For this review, take the finished solid that the model builds, in its own axes (mm). Coordinates: 2 decimals unless noted, no trailing zeros. Write each loop counter-clockwise with the first axis right and the second up, starting at its lowest first coordinate (ties: lowest second). Pieces come first, ordered by that corner, then holes. Notation, with made-up numbers: M 37.5,-4 L 48.5,-4 A14 cw 48.5,2 Z; hole C 49,-20 d4. An arc over 180 degrees is marked long. Return JSON: item names as keys, results as strings.
Autodesk Inventor part; units mm, degrees
ref_plane "YZ Plane" through (0, 0, 0) normal (1, 0, 0) x (0, 1, 0)
ref_plane "XZ Plane" through (0, 0, 0) normal (0, 1, 0) x (-1, 0, 0)
ref_plane "XY Plane" through (0, 0, 0) normal (0, 0, 1) x (1, 0, 0)
sketch "Sketch1" plane through (0, 0, 0) normal (0, 0, 1) x (1, 0, 0)
  line L0 (-52.5, -60) -> (52.5, -60)
  line L1 (52.5, -60) -> (52.5, 60)
  line L2 (52.5, 60) -> (-52.5, 60)
  line L3 (-52.5, 60) -> (-52.5, -60)
  line L4 (-52.5, -60) -> (52.5, 60) construction
  line L5 (52.5, -60) -> (-52.5, 60) construction
  point P0 (0, 0)
  dimension "d0" = 105
  dimension "d1" = 120
extrude "Extrusion1" add sketch "Sketch1" along normal blind 3
sketch "Sketch2" plane through (0, 0, 3) normal (0, 0, 1) x (1, 0, 0)
  circle A0 centre (-47, 55) radius 1.75
  line L0 (-73.5, 0) -> (73.5, 0) construction
  line L1 (0, 84) -> (0, -84) construction
  circle A1 centre (47, 55) radius 1.75
  circle A2 centre (-47, -55) radius 1.75
  circle A3 centre (47, -55) radius 1.75
  point P0 (0, 0)
  dimension "d4" = 3.5
  dimension "d5" = 94
  dimension "d6" = 110
extrude "Extrusion2" cut sketch "Sketch2" against normal blind 3
sketch "Sketch3" plane through (0, 0, 3) normal (0, 0, 1) x (1, 0, 0)
  line L0 (52.5, 60) -> (-52.5, 60) construction
  line L1 (52.5, 60) -> (-52.5, 60) construction
  line L2 (-41, 60) -> (41, 60)
  line L3 (41, 60) -> (41, 15)
  line L4 (41, 15) -> (-41, 15)
  line L5 (-41, 15) -> (-41, 60)
  line L6 (-52.5, 60) -> (-52.5, -60) construction
  line L7 (52.5, -60) -> (52.5, 60) construction
  line L8 (-73.5, 0) -> (73.5, 0)
  line L9 (52.5, -60) -> (-52.5, -60) construction
  line L10 (52.5, -60) -> (-52.5, -60) construction
  line L11 (-41, -60) -> (41, -60)
  line L12 (41, -60) -> (41, -15)
  line L13 (41, -15) -> (-41, -15)
  line L14 (-41, -15) -> (-41, -60)
  point P0 (0, 0)
  dimension "d9" = 15
  dimension "d10" = 82
  dimension "d11" = 11.5
  dimension "d12" = 105
extrude "Extrusion3" cut sketch "Sketch3" against normal blind 3
fillet "Fillet1" radius 2 4 edges at (-41, 15, 1.5) (41, 15, 1.5) (41, -15, 1.5) (-41, -15, 1.5)
fillet "Fillet2" radius 2 8 edges at (41, 60, 1.5) (52.5, 60, 1.5) (-41, 60, 1.5) (-52.5, 60, 1.5) (-52.5, -60, 1.5) (-41, -60, 1.5) (41, -60, 1.5) (52.5, -60, 1.5)
chamfer "Chamfer1" distance 0.75 angle 45 24 edges at (52.5, 0, 3) (51.9142, 59.4142, 3) (46.75, 60, 3) (41.5858, 59.4142, 3) (41, 37.5, 3) (40.4142, 15.5858, 3) (0, 15, 3) (-40.4142, 15.5858, 3) (-41, 37.5, 3) (-41.5858, 59.4142, 3) (-46.75, 60, 3) (-51.9142, 59.4142, 3) (-52.5, 0, 3) (-51.9142, -59.4142, 3) (-46.75, -60, 3) (-41.5858, -59.4142, 3) (-41, -37.5, 3) (-40.4142, -15.5858, 3) (0, -15, 3) (40.4142, -15.5858, 3) (41, -37.5, 3) (41.5858, -59.4142, 3) (46.75, -60, 3) (51.9142, -59.4142, 3)
sketch "Sketch4" plane through (0, 0, 3) normal (0, 0, 1) x (1, 0, 0)
  line L0 (-41, 17) -> (-41, 58)
  arc A0 (-41, 17) -> (-39, 15) centre (-39, 17) ccw
  line L1 (39, 15) -> (-39, 15)
  arc A1 (39, 15) -> (41, 17) centre (39, 17) ccw
  line L2 (41, 58) -> (41, 17)
  arc A2 (43, 60) -> (41, 58) centre (43, 58) ccw
  line L3 (50.5, 60) -> (43, 60)
  arc A3 (52.5, 58) -> (50.5, 60) centre (50.5, 58) ccw
  line L4 (52.5, -58) -> (52.5, 58)
  arc A4 (50.5, -60) -> (52.5, -58) centre (50.5, -58) ccw
  line L5 (43, -60) -> (50.5, -60)
  arc A5 (41, -58) -> (43, -60) centre (43, -58) ccw
  line L6 (41, -17) -> (41, -58)
  arc A6 (41, -17) -> (39, -15) centre (39, -17) ccw
  line L7 (-39, -15) -> (39, -15)
  arc A7 (-39, -15) -> (-41, -17) centre (-39, -17) ccw
  line L8 (-41, -58) -> (-41, -17)
  arc A8 (-43, -60) -> (-41, -58) centre (-43, -58) ccw
  line L9 (-50.5, -60) -> (-43, -60)
  arc A9 (-52.5, -58) -> (-50.5, -60) centre (-50.5, -58) ccw
  line L10 (-52.5, 58) -> (-52.5, -58)
  arc A10 (-50.5, 60) -> (-52.5, 58) centre (-50.5, 58) ccw
  line L11 (-43, 60) -> (-50.5, 60)
  arc A11 (-41, 58) -> (-43, 60) centre (-43, 58) ccw
  circle A12 centre (-47, 55) radius 1.75
  circle A13 centre (47, 55) radius 1.75
  circle A14 centre (47, -55) radius 1.75
  circle A15 centre (-47, -55) radius 1.75
  point P0 (0, 0)
equation "\"d11\" = -0.5 * d10 + 0.5 * d12"
properties part number "BatteryHolderTop"
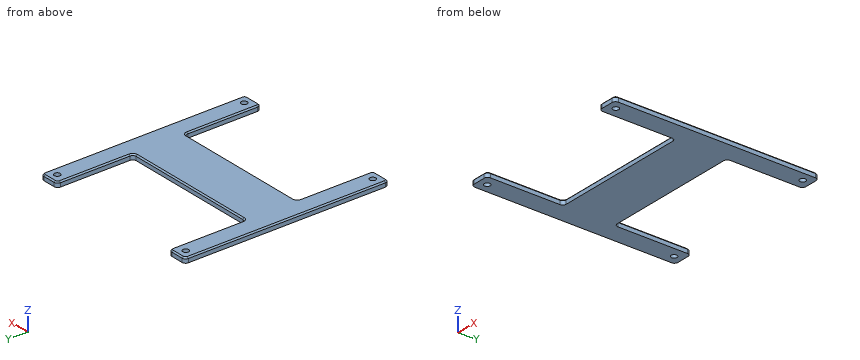
1. Clearance check with flat-ended pins moving along their axes: pin 1 Ø3 at (x, y) = (-47, -55) entering from +Z; pin 2 Ø1.5 at (x, z) = (15, 0.5) entering from +Y; pin 3 Ø1 at (x, z) = (-41.5, 2) entering from -Y; pin 4 Ø1.5 at (x, z) = (-34, 1) entering from -Y. State where each tip first meets the part, or that it passes through.
Checks:
{"pin 1": "through", "pin 2": "y = 15", "pin 3": "y = -59.73", "pin 4": "y = -15"}
2. Wall thickness on L1, parallel to Y at x = -47, z = 0.9; L2, parallel to X at y = -17, z = 2.15; L3, parallel to X at y = -28, z = 2.45: over which ranges is each line inside the solid? List them lowest first. Write a range as from..to.
Checks:
{"L1": "-60..-56.75, -53.25..53.25, 56.75..60", "L2": "-52.5..-41, 41..52.5", "L3": "-52.3..-41.2, 41.2..52.3"}
3. We need section C-C (z = 1.15). State the section outline as (x, y) points.
Checks:
{"outline": "M -52.5,-58 A2 ccw -50.5,-60 L -43,-60 A2 ccw -41,-58 L -41,-17 A2 cw -39,-15 L 39,-15 A2 cw 41,-17 L 41,-58 A2 ccw 43,-60 L 50.5,-60 A2 ccw 52.5,-58 L 52.5,58 A2 ccw 50.5,60 L 43,60 A2 ccw 41,58 L 41,17 A2 cw 39,15 L -39,15 A2 cw -41,17 L -41,58 A2 ccw -43,60 L -50.5,60 A2 ccw -52.5,58 Z; hole C -47,-55 d3.5; hole C -47,55 d3.5; hole C 47,-55 d3.5; hole C 47,55 d3.5"}
4. We need section A-A (y = -37). State the section outline as (x, z) points.
Checks:
{"outline": "M -52.5,0 L -41,0 L -41,2.25 L -41.75,3 L -51.75,3 L -52.5,2.25 Z; M 41,0 L 52.5,0 L 52.5,2.25 L 51.75,3 L 41.75,3 L 41,2.25 Z"}
5. We need section D-D (y = -55). State the section outline as (x, z) points.
Checks:
{"outline": "M -52.5,0 L -48.75,0 L -48.75,3 L -51.75,3 L -52.5,2.25 Z; M -45.25,0 L -41,0 L -41,2.25 L -41.75,3 L -45.25,3 Z; M 41,0 L 45.25,0 L 45.25,3 L 41.75,3 L 41,2.25 Z; M 48.75,0 L 52.5,0 L 52.5,2.25 L 51.75,3 L 48.75,3 Z"}
6. We need section B-B (x = -47). State the section outline as (y, z) points, plus the area to 3 significant figures.
Checks:
{"outline": "M -60,0 L -56.75,0 L -56.75,3 L -59.25,3 L -60,2.25 Z; M -53.25,0 L 53.25,0 L 53.25,3 L -53.25,3 Z; M 56.75,0 L 60,0 L 60,2.25 L 59.25,3 L 56.75,3 Z", "area": "338 mm2"}
